For this review, take the finished solid that the model builds, in its own axes (mm). A direction names the side the tool comes from. Coordinates: 2 decimals unless noted, no trailing zeros. Order: outer loops, then holes, each group sorted by start corner. A loop starts at its lowest first (then second) coordinate and runs counter-clockwise, first axis right, second up. Notation, with made-up numbers: (-11, 20.25) -> (25, 20.25) arc R10 cw to (25, 35.25) -> close; hole circle Ø3 at (-22, -7.5). An arc over 180 degrees is marked (long way). Answer as a JSON object with one key per item and string values. Group by question number.
1) Add section B-B, the plane x = 0. Write out the cut boundary in (y, z), then the cut area to 3 significant figures.
2) Add section A-A, the plane z = 0. Write out the cut boundary in (x, y).
3) Draft analysis for pull direction Z (two halves, no side actions). For faces 3 (the conical face through (9.237, 6.577, -2.909)), 4 (the flat face through (0, 0, 2)), 5 (the flat face through (-2, 4, 0)), state which applies: +Z half, -Z half, draft (parallel to the pull), parting line (faces both ways), or undercut.
4) Wall thickness on L1, parallel to Z at x = 0, y = 6.75; L2, parallel to Z at x = 0, y = 0.9; L3, parallel to X at y = 8, z = 0: over which ranges is each line inside the solid? List them lowest first.
5) For pin 1 (1.5 mm diameter, centred on x = -6.5, y = 4, fed in from -Z); pin 2 (6 mm diameter, centred on x = 8, y = 8.5, fed in from +Z); pin 3 (2 mm diameter, centred on x = 7.5, y = 8, fed in from -Z), all flat-tipped, find the tip position at first contact; note any pin that passes through.
6) Add section D-D, the plane y = 2. Write out the cut boundary in (x, z).
7) Machinability: for faces 1 (the cylindrical face through (-1.216, 2.028, -1.115)), 2 (the cylindrical face through (-0.867, 7.042, 3.905)), which of the approach directions +Z, -Z, +X, -X, +Y, -Y give a long, thin tool a straight path to every point of the face, cutting with its end or side? Answer none if there is none.
8) Add section C-C, the plane y = 6.25. Write out the cut boundary in (x, z), then the cut area to 3 significant figures.
from build123d import *

# Parameters (mm, degrees)
FILLET_1_R = 1


with BuildPart() as part:
    # 草图6 → 旋转1 (revolve)
    with BuildSketch(Plane.XY):
        Polygon((1.65, 0), (1.65, 4), (4, 4), (4, 10), (9, 10), (11, 0), align=None)
    revolve(axis=Axis((0, 0, 0), (0, 1, 0)))

    # 圆角1
    fillet_1_edges = [part.edges().sort_by_distance(p)[0] for p in [
        (-9, 10, 0),
    ]]
    fillet(fillet_1_edges, radius=FILLET_1_R)


solid = part.part
Output values:
{
 "1": {"outline": "(0, -11) -> (9.2, -9.16) arc R1 ccw to (10, -8.18) -> (10, -4) -> (4, -4) -> (4, -1.65) -> (0, -1.65) -> close; (0, 1.65) -> (4, 1.65) -> (4, 4) -> (10, 4) -> (10, 8.18) arc R1 ccw to (9.2, 9.16) -> (0, 11) -> close", "area": "139 mm²"},
 "2": {"outline": "(-11, 0) -> (-1.65, 0) -> (-1.65, 4) -> (-4, 4) -> (-4, 10) -> (-8.18, 10) arc R1 ccw to (-9.16, 9.2) -> close; (1.65, 0) -> (11, 0) -> (9.16, 9.2) arc R1 ccw to (8.18, 10) -> (4, 10) -> (4, 4) -> (1.65, 4) -> close"},
 "3": {"face 3": "parting line", "face 4": "draft", "face 5": "undercut"},
 "4": {"L1": "z = -9.65 to -4, 4 to 9.65", "L2": "z = -10.82 to -1.65, 1.65 to 10.82", "L3": "x = -9.4 to -4, 4 to 9.4"},
 "5": {"pin 1": "stops at z = -8.46", "pin 2": "stops at z = 7.97", "pin 3": "stops at z = -6.83"},
 "6": {"outline": "circle Ø21.2 at (0, 0); hole circle Ø3.3 at (0, 0)"},
 "7": {"face 1": "+Y, -Y", "face 2": "+Y"},
 "8": {"outline": "circle Ø19.5 at (0, 0); hole circle Ø8 at (0, 0)", "area": "248 mm²"}
}
